from build123d import *

# Parameters (mm, degrees)
F0_R     = 11
F1_DEPTH = 7
F2_R     = 8
F3_R     = 8


with BuildPart() as f1:
    # F0 (on Top) → F1 (new body)
    with BuildSketch(Plane.XY):
        with BuildLine():
            ThreePointArc((4.8216833096, -12.0727532097), (10.7629429763, -7.2910258872), (13, 0))
            ThreePointArc((13, 0), (10.7629429763, 7.2910258872), (4.8216833096, 12.0727532097))
            Line((4.8216833096, 12.0727532097), (0, 13))
            Line((0, 13), (-4.8216833096, 12.0727532097))
            ThreePointArc((-4.8216833096, 12.0727532097), (-13, 0), (-4.8216833096, -12.0727532097))
            Line((-4.8216833096, -12.0727532097), (0, -13))
            Line((0, -13), (4.8216833096, -12.0727532097))
        make_face()
        Circle(F0_R, mode=Mode.SUBTRACT)
        with BuildLine():
            ThreePointArc((4.8216833096, 12.0727532097), (10.7629429763, 7.2910258872), (13, 0))
            ThreePointArc((13, 0), (10.7629429763, -7.2910258872), (4.8216833096, -12.0727532097))
            Line((4.8216833096, -12.0727532097), (26, -8))
            ThreePointArc((26, -8), (18, 0), (26, 8))
            Line((26, 8), (4.8216833096, 12.0727532097))
        make_face()
        with BuildLine():
            ThreePointArc((34, 0), (31.6568542495, 5.6568542495), (26, 8))
            ThreePointArc((26, 8), (18, 0), (26, -8))
            ThreePointArc((26, -8), (31.6568542495, -5.6568542495), (34, 0))
        make_face()
        with BuildLine():
            ThreePointArc((-4.8216833096, -12.0727532097), (-13, 0), (-4.8216833096, 12.0727532097))
            Line((-4.8216833096, 12.0727532097), (-26, 8))
            ThreePointArc((-26, 8), (-20.3431457505, 5.6568542495), (-18, 0))
            ThreePointArc((-18, 0), (-20.3431457505, -5.6568542495), (-26, -8))
            Line((-26, -8), (-4.8216833096, -12.0727532097))
        make_face()
        with BuildLine():
            ThreePointArc((-18, 0), (-20.3431457505, 5.6568542495), (-26, 8))
            ThreePointArc((-26, 8), (-34, 0), (-26, -8))
            ThreePointArc((-26, -8), (-20.3431457505, -5.6568542495), (-18, 0))
        make_face()
    extrude(amount=F1_DEPTH)

    # F2
    f2_edges = [f1.edges().sort_by_distance(p)[0] for p in [
        (0, -13, 3.5),
        (0, 13, 3.5),
    ]]
    fillet(f2_edges, radius=F2_R)

    # F3
    f3_edges = [f1.edges().sort_by_distance(p)[0] for p in [
        (-26, -8, 3.5),
        (-26, 8, 3.5),
        (26, 8, 3.5),
        (26, -8, 3.5),
    ]]
    fillet(f3_edges, radius=F3_R)


solid = f1.part
The listing builds one solid part. Answer for the finished solid, in the listing's coordinates (mm). Give positions to 0.01 mm unless a question says otherwise; leave off trailing zeros. Write each loop counter-clockwise with the first axis right and the second up, starting at its lowest first coordinate (ties: lowest second). Pieces come first, ordered by that corner, then holes. Notation, with made-up numbers: (4, 22) -> (25, 22) arc R24 ccw to (25, 60) -> close; hole circle Ø3 at (-37, 22). An arc over 180 degrees is marked (long way). Use a Markdown table: item, result.
(1) Find the intervals of material crossed by probe 1 along Y at (x, z) = (0, 4.75); probe 2 along Y at (x, z) = (8, 4.25); probe 3 along X at (y, z) = (-5.25, 3), in increasing order. Write a range as from..to.
Return value:
| item | result |
|---|---|
| probe 1 | -12.85..-11, 11..12.85 |
| probe 2 | -11.46..-7.55, 7.55..11.46 |
| probe 3 | -32.04..-9.67, 9.67..32.04 |
(2) Determine the mould class of faces 1 (the cylindrical face through (-2.38, -10.74, 3.45)), 2 (the cylindrical face through (0.021, -12.853, 3.549)), 3 (the flat face through (-0.5, -11.2, 0)) for opening direction X: released by +X, released by -X, zero draft, split by the parting line, or undercut.
Return value:
| item | result |
|---|---|
| face 1 | undercut |
| face 2 | split by the parting line |
| face 3 | zero draft |
(3) Section D-D, the plane x = -22 is taken. Determine the outline of the cut face in (y, z), then the cut area to 3 significant figures.
Return value:
| item | result |
|---|---|
| outline | (-8.77, 0) -> (8.77, 0) -> (8.77, 7) -> (-8.77, 7) -> close |
| area | 123 mm2 |
(4) Flat-ended cylindrical pins translate along their axes: P1, Ø1.5, axis at y = -5.5, z = 2.5, coming from the +X side; P2, Ø6, axis at x = -23, y = 2.5, coming from the -Z side. Find the tip coordinate at first contact, or state that the pin passes through.
Return value:
| item | result |
|---|---|
| P1 | x = 32.44 |
| P2 | z = 0 |
(5) Section C-C, the plane x = 9 is taken. Determine the outline of the cut face in (y, z).
Return value:
| item | result |
|---|---|
| outline | (-11.27, 0) -> (-6.32, 0) -> (-6.32, 7) -> (-11.27, 7) -> close; (6.32, 0) -> (11.27, 0) -> (11.27, 7) -> (6.32, 7) -> close |
(6) Section A-A, the plane z = 2.25 is taken. Determine the outline of the cut face in (x, y), then the cut area to 3 significant figures.
Return value:
| item | result |
|---|---|
| outline | (-26.45, -7.99) arc R8 cw to (-25.38, -8.12) -> (-1.51, -12.71) arc R8 ccw to (1.51, -12.71) -> (25.38, -8.12) arc R8 cw to (26.45, -7.99) arc R8 ccw to (26.45, 7.99) arc R8 cw to (25.38, 8.12) -> (1.51, 12.71) arc R8 ccw to (-1.51, 12.71) -> (-25.38, 8.12) arc R8 cw to (-26.45, 7.99) arc R8 ccw to start; hole circle Ø22 at (0, 0) |
| area | 913 mm2 |
(7) Section B-B, the plane y = -9 is taken. Determine the outline of the cut face in (x, z).
Return value:
| item | result |
|---|---|
| outline | (-20.8, 0) -> (-6.32, 0) -> (-6.32, 7) -> (-20.8, 7) -> close; (6.32, 0) -> (20.8, 0) -> (20.8, 7) -> (6.32, 7) -> close |
